Read the model definition and answer for the solid it produces. Units are mm, in the model's axes. A direction names the side the tool comes from. Give positions to 0.01 mm unless a question says otherwise; leave off trailing zeros. Order: outer loops, then holes, each group sorted by start corner. A loop starts at its lowest first (then second) coordinate and runs counter-clockwise, first axis right, second up. Notation, with made-up numbers: (4.25, 36.5) -> (24.25, 36.5) arc R15 ccw to (24.25, 43.5) -> close; hole circle Ø11 at (30.5, -18.75). An arc over 180 degrees is marked (long way). Use one line per item in the form item = value.
```python
from build123d import *

# Parameters (mm, degrees)
F1_DEPTH = 13
F2_DEPTH = 36
F3_DEPTH = 3
F4_R     = 2
F6_D     = 12
F6_DEPTH = 12
F6_TIP   = 3.6051637142
F7_ANGLE = 180


with BuildPart() as f1:
    # F0 (on Top) → F1 (new body)
    with BuildSketch(Plane.XY):
        with BuildLine():
            ThreePointArc((29.5146428337, 10), (31.1042871443, 10.6969432761), (32.4494111737, 11.7939119674))
            Line((32.4494111737, 11.7939119674), (108.2332133573, 87.2420420008))
            ThreePointArc((108.2332133573, 87.2420420008), (109.5407255907, 89.1918380595), (110, 91.4940891162))
            Line((110, 91.4940891162), (110, 99.372583002))
            ThreePointArc((110, 99.372583002), (109.5432771951, 101.6686835962), (108.2426406871, 103.6152236891))
            Line((108.2426406871, 103.6152236891), (103.6152236891, 108.2426406871))
            ThreePointArc((103.6152236891, 108.2426406871), (101.6686835962, 109.5432771951), (99.372583002, 110))
            Line((99.372583002, 110), (12, 110))
            ThreePointArc((12, 110), (10.5857864376, 109.4142135624), (10, 108))
            Line((10, 108), (10, 20.627416998))
            ThreePointArc((10, 20.627416998), (10.4567228049, 18.3313164038), (11.7573593129, 16.3847763109))
            Line((11.7573593129, 16.3847763109), (16.3847763109, 11.7573593129))
            ThreePointArc((16.3847763109, 11.7573593129), (18.3313164038, 10.4567228049), (20.627416998, 10))
            Line((20.627416998, 10), (29.5146428337, 10))
        make_face()
        with BuildLine():
            ThreePointArc((91.8982009854, 95.2846255964), (95.433726402, 95.2767779765), (95.4258783418, 91.7412525609))
            Line((95.4258783418, 91.7412525609), (28.1017990146, 24.7153744036))
            ThreePointArc((28.1017990146, 24.7153744036), (24.5662740393, 24.7232224629), (24.5741216582, 28.2587474391))
            Line((24.5741216582, 28.2587474391), (47.6067560594, 51.1893624946))
            Line((47.6067560594, 51.1893624946), (45.5464457109, 53.2588392572))
            ThreePointArc((45.5464457109, 53.2588392572), (45.506735129, 57.5600725399), (49.8074020179, 57.4797669158))
            Line((49.8074020179, 57.4797669158), (51.794521287, 55.3585786904))
            Line((51.794521287, 55.3585786904), (91.8982009854, 95.2846255964))
        make_face(mode=Mode.SUBTRACT)
    extrude(amount=F1_DEPTH)

    # F0 (on Top) → F2 (join)
    with BuildSketch(Plane.XY):
        Polygon((0, 14), (14, 0), (114, 0), (120, 6), (120, 106), (106, 120), (6, 120), (0, 114), align=None)
        with BuildLine():
            Line((108.2332133573, 87.2420420008), (32.4494111737, 11.7939119674))
            ThreePointArc((32.4494111737, 11.7939119674), (31.1042871443, 10.6969432761), (29.5146428337, 10))
            Line((29.5146428337, 10), (20.627416998, 10))
            ThreePointArc((20.627416998, 10), (18.3313164038, 10.4567228049), (16.3847763109, 11.7573593129))
            Line((16.3847763109, 11.7573593129), (11.7573593129, 16.3847763109))
            ThreePointArc((11.7573593129, 16.3847763109), (10.4567228049, 18.3313164038), (10, 20.627416998))
            Line((10, 20.627416998), (10, 108))
            ThreePointArc((10, 108), (10.5857864376, 109.4142135624), (12, 110))
            Line((12, 110), (99.372583002, 110))
            ThreePointArc((99.372583002, 110), (101.6686835962, 109.5432771951), (103.6152236891, 108.2426406871))
            Line((103.6152236891, 108.2426406871), (108.2426406871, 103.6152236891))
            ThreePointArc((108.2426406871, 103.6152236891), (109.5432771951, 101.6686835962), (110, 99.372583002))
            Line((110, 99.372583002), (110, 91.4940891162))
            ThreePointArc((110, 91.4940891162), (109.5407255907, 89.1918380595), (108.2332133573, 87.2420420008))
        make_face(mode=Mode.SUBTRACT)
    extrude(amount=F2_DEPTH)

    # F0 (on Top) → F3 (join)
    with BuildSketch(Plane.XY):
        with BuildLine():
            Line((49.8360901626, 53.4088221213), (51.794521287, 55.3585786904))
            Line((51.794521287, 55.3585786904), (49.8074020179, 57.4797669158))
            ThreePointArc((49.8074020179, 57.4797669158), (45.506735129, 57.5600725399), (45.5464457109, 53.2588392572))
            Line((45.5464457109, 53.2588392572), (47.6067560594, 51.1893624946))
            Line((47.6067560594, 51.1893624946), (49.6280971878, 53.201750418))
            Line((49.6280971878, 53.201750418), (49.8360901626, 53.4088221213))
        make_face()
    extrude(amount=F3_DEPTH)

    # F4
    f4_edges = [f1.edges().sort_by_distance(p)[0] for p in [
        (56, 120, 0),
        (106, 120, 18),
        (120, 106, 18),
        (120, 56, 0),
        (113, 113, 0),
        (117, 3, 0),
        (114, 0, 18),
        (120, 6, 18),
        (64, 0, 0),
        (14, 0, 18),
        (7, 7, 0),
        (0, 14, 18),
        (0, 64, 0),
        (3, 117, 0),
        (0, 114, 18),
        (6, 120, 18),
    ]]
    fillet(f4_edges, radius=F4_R)

    # F6
    with Locations(Plane(origin=(0, 0, 0), x_dir=(0, -1, 0), z_dir=(-1, 0, 0))):
        with Locations((-89, 19.5)):
            Hole(F6_D / 2, depth=F6_DEPTH)
            with Locations((0, 0, -(F6_DEPTH + F6_TIP / 2))):  # 118° drill point
                Cone(0, F6_D / 2, F6_TIP, mode=Mode.SUBTRACT)


with BuildPart() as f1_1:
    # F7: moved
    add(f1.part.rotate(Axis((64, 2, 0), (-1, 0, 0)), F7_ANGLE))


solid = f1_1.part
```
Item 1: Given pin 1 Ø12 at (x, y) = (18.5, -53) entering from -Z; pin 2 Ø1 at (y, z) = (-8, -16) entering from -X, each flat-ended and moving along its own axis, determine where each tip first touches the part or whether it passes through.
Checks:
pin_1 = -13
pin_2 = 1.5
Item 2: Determine the mould class of faces 4 (the cylindrical face through (3.39, -112.54, -0.57)), 5 (the flat face through (63, 4, -19)), 6 (the flat face through (48, -68, -13)) for opening direction Y: +Y half, -Y half, draft (parallel to the pull), parting line (faces both ways), or undercut.
Checks:
face_4 = -Y half
face_5 = +Y half
face_6 = undercut
Item 3: Straight lines are drawn through the part: L1, parallel to Z at x = 8, y = -85; L2, parallel to Y at x = 21.5, z = -20; L3, parallel to Z at x = 16.5, y = -37. For each, find the intervals that lie inside material, in ascending order. Write a range as from..to.
Checks:
L1 = -36..-25.5, -13.5..0
L2 = -116..-106, -6..4
L3 = -13..0
Item 4: Which of the six approach directions +Z, -Z, +X, -X, +Y, -Y give full straight-line access (tool end or side, diameter ignored) to faces 1 (the cylindrical face through (101.638, -105.556, -24.339)), 2 (the flat face through (113, -109, -19)), 3 (the cylindrical face through (5.07, -79.006, -19.764))?
Checks:
face_1 = -Z
face_2 = +Z, -Z, +X, -Y
face_3 = -X
Item 5: The part is cut by section C-C on x = 90.5. Give the vertices of the cut face in (y, z).
Checks:
outline = (-116, -36) -> (-106, -36) -> (-106, -13) -> (-89.89, -13) -> (-89.89, 0) -> (-114, 0) arc R2 ccw to (-116, -2) -> close; (-82.84, -13) -> (-65.59, -13) -> (-65.59, -36) -> (4, -36) -> (4, -2) arc R2 ccw to (2, 0) -> (-82.84, 0) -> close
Item 6: The part is cut by section B-B on y = -57.5. Give the vertices of the cut face in (x, z), and give its area (3 significant figures).
Checks:
outline = (0, -36) -> (10, -36) -> (10, -13) -> (57.96, -13) -> (57.96, 0) -> (2, 0) arc R2 ccw to (0, -2) -> close; (65.05, -13) -> (82.38, -13) -> (82.38, -36) -> (120, -36) -> (120, -2) arc R2 ccw to (118, 0) -> (65.05, 0) -> close
area = 2,560 mm²
